CAD build for the part. Positions are in the model's coordinates, mm. Round coordinates to 2 decimals unless told otherwise and drop trailing zeros. Order: outer loops, then holes, each group sorted by start corner. A loop starts at its lowest first (then second) coordinate and runs counter-clockwise, first axis right, second up. Notation, with made-up numbers: (58.25, 44.5) - (101.25, 44.5) arc R20 ccw to (101.25, 52.5) - close; hole circle Ø2 at (33.5, 44). An arc over 180 degrees is marked (long way). Use one line per item in the form item = value. Start each with the question number.
from build123d import *

# Parameters (mm, degrees)
BOSS_EXTRUDE1_DEPTH = 6.35
SKETCH2_R           = 2.4638
CUT_EXTRUDE1_DEPTH  = 7.35
LPATTERN1_COUNT     = 6
LPATTERN1_PITCH     = 50.8
SKETCH3_R           = 2.4638
CUT_EXTRUDE2_DEPTH  = 7.35
LPATTERN2_COUNT     = 4
LPATTERN2_PITCH     = 101.6
SKETCH4_R           = 3.3655
CUT_EXTRUDE3_DEPTH  = 7.35
FILLET1_R           = 6.35


with BuildPart() as part:
    # Sketch1 → Boss-Extrude1 (new body)
    with BuildSketch(Plane.XY):
        Polygon((-463.55, -82.55), (-463.55, 0), (463.55, 0), (463.55, -82.55), (247.65, -82.55), (247.65, -298.45), (-247.65, -298.45), (-247.65, -82.55), align=None)
    extrude(amount=BOSS_EXTRUDE1_DEPTH)

    # Sketch2 → Cut-Extrude1 (cut, through all)
    with BuildSketch(Plane.XY.offset(6.35)):
        with Locations((127, -9.525)):
            Circle(SKETCH2_R)
    cut_extrude1 = extrude(amount=-CUT_EXTRUDE1_DEPTH, mode=Mode.SUBTRACT)

    # LPattern1: Cut-Extrude1 ×6
    with Locations(*[(-i * LPATTERN1_PITCH, 0, 0) for i in range(1, LPATTERN1_COUNT)]):
        add(cut_extrude1, mode=Mode.SUBTRACT)

    # Sketch3 → Cut-Extrude2 (cut, through all)
    with BuildSketch(Plane.XY.offset(6.35)):
        with Locations((-152.4, -273.05)):
            Circle(SKETCH3_R)
    cut_extrude2 = extrude(amount=-CUT_EXTRUDE2_DEPTH, mode=Mode.SUBTRACT)

    # LPattern2: Cut-Extrude2 ×4
    with Locations(*[(i * LPATTERN2_PITCH, 0, 0) for i in range(1, LPATTERN2_COUNT)]):
        add(cut_extrude2, mode=Mode.SUBTRACT)

    # Sketch4 → Cut-Extrude3 (cut, through all)
    with BuildSketch(Plane.XY.offset(6.35)):
        with Locations((-24.13, -139.7)):
            Circle(SKETCH4_R)
        with Locations((24.13, -139.7)):
            Circle(SKETCH4_R)
    extrude(amount=-CUT_EXTRUDE3_DEPTH, mode=Mode.SUBTRACT)

    # Fillet1
    fillet1_edges = [part.edges().sort_by_distance(p)[0] for p in [
        (-463.55, -82.55, 3.175),
        (-463.55, 0, 3.175),
        (463.55, 0, 3.175),
        (463.55, -82.55, 3.175),
        (247.65, -82.55, 3.175),
        (247.65, -298.45, 3.175),
        (-247.65, -298.45, 3.175),
        (-247.65, -82.55, 3.175),
    ]]
    fillet(fillet1_edges, radius=FILLET1_R)


solid = part.part
(1) Flat gauge pins, fed straight in: P1, Ø3, axis at x = 405, z = 4.5, coming from the -Y side; P2, Ø4, axis at x = -50.8, y = -273.05, coming from the +Z side; P3, Ø3, axis at y = -204, z = 4.5, coming from the +X side; P4, Ø1.9, axis at y = -230.5, z = 4, coming from the -X side. Where does each tip first touch, or does it go through?
(2) Slice it at C-C (x = 362.5). Give the cut face in (y, z), and give its area (3 significant figures).
(3) Wall check: line 1 (X direction, y = -273.05, z = 5); line 2 (Y direction, x = -127, z = 3.5); line 3 (Y direction, x = 152.4, z = 5). Give the ranges that are in metal, low to high. Write a range as [from, to].
(4) Slice it at B-B (y = -255). Give the cut face in (x, z).
(5) Slice it at A-A (z = 4.75). Give the number of separate pieces and of enclosed holes in the cut face, and give its area (3 significant figures).
Results list:
q1.P1 = -82.55
q1.P2 = through
q1.P3 = 247.65
q1.P4 = -247.65
q2.outline = (-82.55, 0) - (0, 0) - (0, 6.35) - (-82.55, 6.35) - close
q2.area = 524 mm²
q3.line_1 = [-247.65, -154.86], [-149.94, -53.26], [-48.34, 48.34], [53.26, 149.94], [154.86, 247.65]
q3.line_2 = [-298.45, -11.99], [-7.06, 0]
q3.line_3 = [-298.45, -275.51], [-270.59, 0]
q4.outline = (-247.65, 0) - (247.65, 0) - (247.65, 6.35) - (-247.65, 6.35) - close
q5.separate_pieces = 1
q5.enclosed_holes = 12
q5.area = 183,000 mm²
